For this review, use the dimensioned drawing (mm, ordinates from the lowest corner) and the shaded views. Round coordinates to 2 decimals unless told otherwise and drop trailing zeros. Write each loop counter-clockwise with the first axis right and the second up, starting at its lowest first coordinate (ties: lowest second). Pieces come first, ordered by that corner, then holes. Notation, with made-up numbers: M 8.25,86 L 14.25,86 A23 cw 14.25,103 Z; hole C 80.25,53 d9. An arc over 180 degrees is marked long. Use CSV: the item, a comma, the result in double quotes.
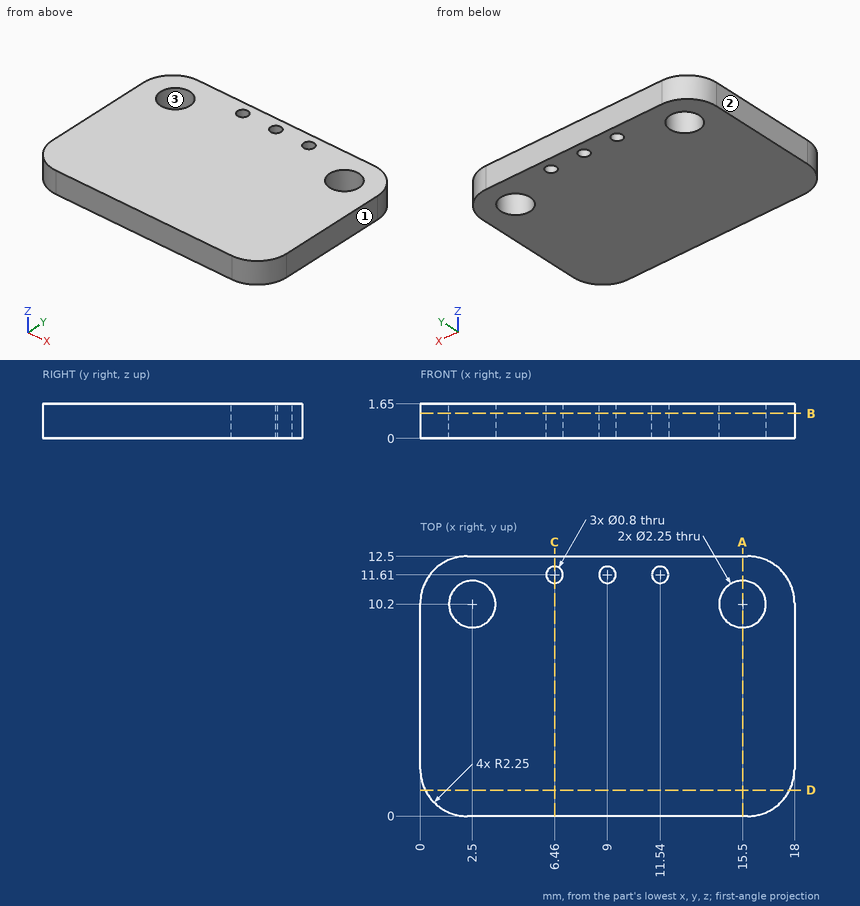
1) Add section B-B on z = 1.2. Write out the cut boundary in (x, y) (3 decimals).
Answers:
outline,"M 0,2.25 A2.25 ccw 2.25,0 L 15.75,0 A2.25 ccw 18,2.25 L 18,10.25 A2.25 ccw 15.75,12.5 L 2.25,12.5 A2.25 ccw 0,10.25 Z; hole C 2.5,10.2 d2.25; hole C 6.46,11.61 d0.8; hole C 9,11.61 d0.8; hole C 11.54,11.61 d0.8; hole C 15.5,10.2 d2.25"
2) The part is to be moulded in two halves that separate along X. For the marked faces 1, 2 and 3, say which applies: released by +X, released by -X, zero draft, split by the parting line, or undercut.
Answers:
face 1,"released by +X"
face 2,"released by -X"
face 3,"undercut"
3) Wall thickness on line 1 along Y through (x, z) = (6.46, 1.15); line 2 along Y through (x, z) = (2.5, 0.85) (3 decimals); line 3 along X through (y, z) = (1.75, 1.5): over which ranges is each line inside the solid? List them lowest first. Write a range as [from, to].
Answers:
line 1,"[0, 11.21], [12.01, 12.5]"
line 2,"[0, 9.075], [11.325, 12.5]"
line 3,"[0.06, 17.94]"
4) Add section C-C on x = 6.46. Write out the cut boundary in (y, z).
Answers:
outline,"M 0,0 L 11.21,0 L 11.21,1.65 L 0,1.65 Z; M 12.01,0 L 12.5,0 L 12.5,1.65 L 12.01,1.65 Z"
5) Add section D-D on y = 1.25. Write out the cut boundary in (x, z).
Answers:
outline,"M 0.23,0 L 17.77,0 L 17.77,1.65 L 0.23,1.65 Z"
6) Add section A-A on x = 15.5. Write out the cut boundary in (y, z) (3 decimals), then the cut area to 3 significant figures.
Answers:
outline,"M 0,0 L 9.075,0 L 9.075,1.65 L 0,1.65 Z; M 11.325,0 L 12.5,0 L 12.5,1.65 L 11.325,1.65 Z"
area,"16.9 mm²"
